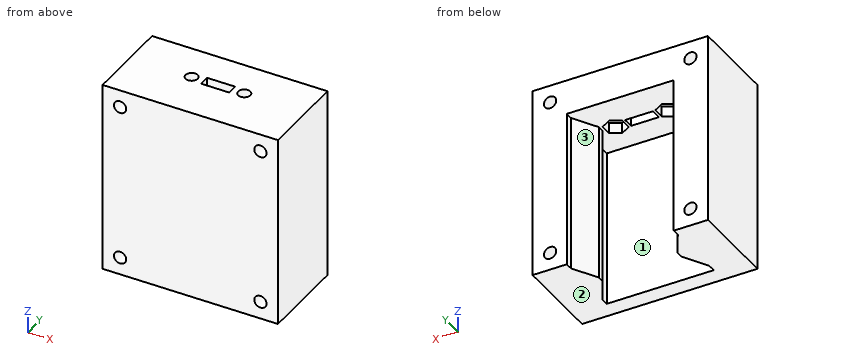
from build123d import *

# Parameters (mm, degrees)
SCHIZZO1_W                   = 50
SCHIZZO1_H                   = 25
SCHIZZO1_R                   = 1.75
SCHIZZO1_W_2                 = 8
SCHIZZO1_H_2                 = 3
ESTRUSIONE_ESTRUSIONE1_DEPTH = 10
ESTRUSIONE_ESTRUSIONE2_DEPTH = 45
TAGLIO_ESTRUSIONE1_DEPTH     = 3
SCHIZZO4_R                   = 1.75
TAGLIO_ESTRUSIONE2_DEPTH     = 58.227615711


with BuildPart() as part:
    # Schizzo1 → Estrusione-Estrusione1 (new body)
    with BuildSketch(Plane.XY):
        Rectangle(SCHIZZO1_W, SCHIZZO1_H)
        with Locations((-7.5, 1.5)):
            Circle(SCHIZZO1_R, mode=Mode.SUBTRACT)
        with Locations((7.5, 1.5)):
            Circle(SCHIZZO1_R, mode=Mode.SUBTRACT)
        with Locations((0, 1.5)):
            Rectangle(SCHIZZO1_W_2, SCHIZZO1_H_2, mode=Mode.SUBTRACT)
    extrude(amount=ESTRUSIONE_ESTRUSIONE1_DEPTH)

    # Schizzo2 → Estrusione-Estrusione2 (add)
    with BuildSketch(Plane(origin=(0, 0, 0), x_dir=(-1, 0, 0), z_dir=(0, 0, -1))):
        Polygon((-15.241451884, 12.5), (-25, 12.5), (-25, -12.5), (25, -12.5), (25, 12.5), (15.241451884, 12.5), (15.241451884, 10.446410162), (11.2, 3.446410162), (11.2, 1.553589838), (15.241451884, -5.446410162), (15.241451884, -7.7), (0, -7.7), (-15.241451884, -7.7), (-15.241451884, -5.446410162), (-11.2, 1.553589838), (-11.2, 3.446410162), (-15.241451884, 10.446410162), align=None)
    extrude(amount=ESTRUSIONE_ESTRUSIONE2_DEPTH)

    # Schizzo3 → Taglio-Estrusione1 (cut)
    with BuildSketch(Plane(origin=(0, 0, 0), x_dir=(-1, 0, 0), z_dir=(0, 0, -1))):
        Polygon((-7.5, 4.75), (-10.314582562, 3.125), (-10.314582562, -0.125), (-7.5, -1.75), (-4.685417438, -0.125), (-4.685417438, 3.125), align=None)
        Polygon((7.5, 4.75), (4.685417438, 3.125), (4.685417438, -0.125), (7.5, -1.75), (10.314582562, -0.125), (10.314582562, 3.125), align=None)
    extrude(amount=-TAGLIO_ESTRUSIONE1_DEPTH, mode=Mode.SUBTRACT)

    # Schizzo4 → Taglio-Estrusione2 (cut, through all)
    with BuildSketch(Plane(origin=(0, 12.5, 0), x_dir=(1, 0, 0), z_dir=(0, 1, 0))):
        with Locations(Location((-20, -5, 0), (0, 0, 180))):
            Circle(SCHIZZO4_R)
        with Locations(Location((-20, 40, 0), (0, 0, 180))):
            Circle(SCHIZZO4_R)
        with Locations(Location((20, 40, 0), (0, 0, 180))):
            Circle(SCHIZZO4_R)
        with Locations(Location((20, -5, 0), (0, 0, 180))):
            Circle(SCHIZZO4_R)
    extrude(amount=-TAGLIO_ESTRUSIONE2_DEPTH, mode=Mode.SUBTRACT)


solid = part.part
Geometry check sheet. Reference: the model listing, model coordinates, mm. Face numbers are marked on the shaded views. A direction names the side the tool comes from. Round coordinates to 2 decimals unless told otherwise and drop trailing zeros. Order: outer loops, then holes, each group sorted by start corner. A loop starts at its lowest first (then second) coordinate and runs counter-clockwise, first axis right, second up. Notation, with made-up numbers: M 23.25,35 L 75.25,35 A11 ccw 75.25,41 Z; hole C 16.5,-10.75 d2. An arc over 180 degrees is marked long. Answer in a Markdown table with one row per item. Add a question column.
Item 1: Depth check by flat-ended pin: pin 1 Ø3 at (x, y) = (9, 7) entering from -Z; pin 2 Ø3 at (x, y) = (-7.5, 1.5) entering from +Z; pin 3 Ø9 at (x, z) = (4.5, -19) entering from +Y. Enter the tip coordinate at first touch or a pass-through.
Item 2: Sectioned sample at D-D, the plane x = -3. Enter the section's corners in (y, z), plus the area to 3 significant figures.
Item 3: Sectioned sample at A-A, the plane x = -20. Enter the section's corners in (y, z), plus the area to 3 significant figures.
Item 4: Set-up check for the marked faces 1, 2 and 3: record each of +Z, -Z, +X, -X, +Y, -Y from which the full face is reachable in a straight line by a thin tool's end or side.
Item 5: Sectioned sample at C-C, the plane y = 9. Enter the section's corners in (x, z).
Item 6: Sectioned sample at B-B, the plane z = -40. Enter the section's corners in (x, y).
Item 7: Material ranges on L1, parallel to Z at x = 20, y = 0.5; L2, parallel to X at y = 1.5, z = 8; L3, parallel to X at y = 10.5, z = -0.5, recorded low to high. Write a range as [from, to].
Filled in:
| question | item | result |
|---|---|---|
| 1 | pin 1 | stops at z = 0 |
| 1 | pin 2 | passes through |
| 1 | pin 3 | stops at y = -7.7 |
| 2 | outline | M -12.5,-45 L -7.7,-45 L -7.7,0 L 0,0 L 0,10 L -12.5,10 Z; M 3,0 L 12.5,0 L 12.5,10 L 3,10 Z |
| 2 | area | 436 mm² |
| 3 | outline | M -12.5,-45 L 12.5,-45 L 12.5,-41.75 L -12.5,-41.75 Z; M -12.5,-38.25 L 12.5,-38.25 L 12.5,3.25 L -12.5,3.25 Z; M -12.5,6.75 L 12.5,6.75 L 12.5,10 L -12.5,10 Z |
| 3 | area | 1,200 mm² |
| 4 | face 1 | -Z |
| 4 | face 2 | -Z, +X, -X, +Y, -Y |
| 4 | face 3 | -Z, +Y |
| 5 | outline | M -25,-45 L -14.41,-45 L -14.41,0 L 14.41,0 L 14.41,-45 L 25,-45 L 25,10 L -25,10 Z; hole C -20,-40 d3.5; hole C -20,5 d3.5; hole C 20,-40 d3.5; hole C 20,5 d3.5 |
| 6 | outline | M -25,-12.5 L -21.75,-12.5 L -21.75,12.5 L -25,12.5 Z; M -18.25,-12.5 L 18.25,-12.5 L 18.25,12.5 L 15.24,12.5 L 15.24,10.45 L 11.2,3.45 L 11.2,1.55 L 15.24,-5.45 L 15.24,-7.7 L -15.24,-7.7 L -15.24,-5.45 L -11.2,1.55 L -11.2,3.45 L -15.24,10.45 L -15.24,12.5 L -18.25,12.5 Z; M 21.75,-12.5 L 25,-12.5 L 25,12.5 L 21.75,12.5 Z |
| 7 | L1 | z = [-45, -41.75], [-38.25, 3.25], [6.75, 10] |
| 7 | L2 | x = [-25, -9.25], [-5.75, -4], [4, 5.75], [9.25, 25] |
| 7 | L3 | x = [-25, -15.24], [15.24, 25] |
